Check sheet for the modelled part. Datum: model origin and axes. Units: mm. A direction names the side the tool comes from. Round coordinates to 2 decimals unless told otherwise and drop trailing zeros. Order: outer loops, then holes, each group sorted by start corner. A loop starts at its lowest first (then second) coordinate and runs counter-clockwise, first axis right, second up. Notation, with made-up numbers: (89, 59) -> (108, 59) arc R18 cw to (108, 83) -> close; hole circle Ø5 at (79, 5). An arc over 180 degrees is marked (long way). Answer in a Markdown table with one row per item.
from build123d import *

# Parameters (mm, degrees)
BOSS_EXTRUDE1_DEPTH = 15.875
SKETCH2_R           = 1.27
CUT_EXTRUDE1_DEPTH  = 57.969799236
SKETCH3_R           = 3.81
CUT_EXTRUDE2_DEPTH  = 4.1275


with BuildPart() as part:
    # Sketch1 → Boss-Extrude1 (new body)
    with BuildSketch(Plane(origin=(0, 0, 0), x_dir=(1, 0, 0), z_dir=(0, 1, 0))):
        with BuildLine():
            Line((48.26, 0), (2.54, 0))
            ThreePointArc((2.54, 0), (0.743948776, -0.743948776), (0, -2.54))
            Line((0, -2.54), (0, -20.32))
            Line((0, -20.32), (12.4079, -20.32))
            ThreePointArc((12.4079, -20.32), (25.4, -7.3279), (38.3921, -20.32))
            Line((38.3921, -20.32), (50.8, -20.32))
            Line((50.8, -20.32), (50.8, -2.54))
            ThreePointArc((50.8, -2.54), (50.056051224, -0.743948776), (48.26, 0))
        make_face()
    extrude(amount=BOSS_EXTRUDE1_DEPTH)

    # Sketch2 → Cut-Extrude1 (cut, through all)
    with BuildSketch(Plane.XY.offset(20.32)):
        with Locations((6.3119, 7.9375)):
            Circle(SKETCH2_R)
        with Locations((44.6024, 7.9375)):
            Circle(SKETCH2_R)
    extrude(amount=-CUT_EXTRUDE1_DEPTH, mode=Mode.SUBTRACT)

    # Sketch3 → Cut-Extrude2 (cut)
    with BuildSketch(Plane(origin=(0, 0, 0), x_dir=(-1, 0, 0), z_dir=(0, 0, -1))):
        with Locations((-44.6024, 7.9375)):
            Circle(SKETCH3_R)
        with Locations((-6.3119, 7.9375)):
            Circle(SKETCH3_R)
    extrude(amount=-CUT_EXTRUDE2_DEPTH, mode=Mode.SUBTRACT)


solid = part.part
Item 1: Depth check by flat-ended pin: P1, Ø2.5, axis at x = 5.5, y = 8.5, coming from the -Z side; P2, Ø3, axis at x = 16, y = 4, coming from the +Z side. Enter the tip coordinate at first touch or a pass-through.
Result sheet:
| item | result |
|---|---|
| P1 | stops at z = 4.13 |
| P2 | stops at z = 13.25 |
Item 2: Cross-section at C-C (z = 15). Record the boundary of the cut face in (x, y) (1 decimal).
Result sheet:
| item | result |
|---|---|
| outline | (0, 0) -> (13.5, 0) -> (13.5, 15.9) -> (0, 15.9) -> close; (37.3, 0) -> (50.8, 0) -> (50.8, 15.9) -> (37.3, 15.9) -> close; hole circle Ø2.5 at (6.3, 7.9); hole circle Ø2.5 at (44.6, 7.9) |
Item 3: Cross-section at D-D (x = 25.4). Record the boundary of the cut face in (y, z) (3 decimals).
Result sheet:
| item | result |
|---|---|
| outline | (0, 0) -> (15.875, 0) -> (15.875, 7.328) -> (0, 7.328) -> close |
Item 4: Set-up check for faces 5 (the cylindrical face through (6.808, 11.715, 2.035)), 6 (the flat face through (25, 15.875, 6)): record each of +Z, -Z, +X, -X, +Y, -Y from which the full face is reachable in a straight line by a thin tool's end or side.
Result sheet:
| item | result |
|---|---|
| face 5 | -Z |
| face 6 | +Z, -Z, +X, -X, +Y |
Item 5: Cross-section at A-A (z = 8.75). Record the boundary of the cut face in (x, y) (1 decimal), and give its area (3 significant figures).
Result sheet:
| item | result |
|---|---|
| outline | (0, 0) -> (19.5, 0) -> (19.5, 15.9) -> (0, 15.9) -> close; (31.3, 0) -> (50.8, 0) -> (50.8, 15.9) -> (31.3, 15.9) -> close; hole circle Ø2.5 at (6.3, 7.9); hole circle Ø2.5 at (44.6, 7.9) |
| area | 609 mm^2 |
Item 6: Mould release check, pull along X, two halves, no side actions. Record for faces 1 (the flat face through (4.7, 7.8, 20.32)), 2 (the cylindrical face through (0.764, 7.826, 0.724)), 3 (the cylindrical face through (45.776, 7.451, 12.337)), 4 (the flat face through (50.8, 8, 12)): pulls with the +X half, pulls with the -X half, needs draft (parallel to the pull), parting line crosses it, or undercut.
Result sheet:
| item | result |
|---|---|
| face 1 | needs draft |
| face 2 | pulls with the -X half |
| face 3 | undercut |
| face 4 | pulls with the +X half |
Item 7: Cross-section at B-B (y = 13.5). Record the boundary of the cut face in (x, z).
Result sheet:
| item | result |
|---|---|
| outline | (0, 2.54) arc R2.54 ccw to (2.54, 0) -> (48.26, 0) arc R2.54 ccw to (50.8, 2.54) -> (50.8, 20.32) -> (38.39, 20.32) arc R12.99 cw to (12.41, 20.32) -> (0, 20.32) -> close |
Item 8: Scan lines: line 1 (X direction, y = 9, z = 4); line 2 (X direction, y = 7.5, z = 14.5); line 3 (X direction, y = 13, z = 18). Record each from-to range of solid material in increasing order. Write a range as [from, to].
Result sheet:
| item | result |
|---|---|
| line 1 | x = [0, 2.65], [9.97, 40.94], [48.26, 50.8] |
| line 2 | x = [0, 5.12], [7.5, 13.78], [37.02, 43.41], [45.79, 50.8] |
| line 3 | x = [0, 12.62], [38.18, 50.8] |
